from build123d import *

# Parameters (mm, degrees)
BOSS_EXTRU_1_START = -10
BOSS_EXTRU_1_DEPTH = 19
CHANFREIN1_SIZE    = 1.5


with BuildPart() as part:
    # Esquisse1 → Révolution1 (revolve)
    with BuildSketch(Plane.XY, mode=Mode.PRIVATE) as r_volution1_sk:
        Polygon((33, 0), (33, 35), (36, 41), (38.5, 41), (38.5, 42.25), (35.227457514, 42.25), (31.75, 35.295084972), (31.75, 0), align=None)
    revolve(r_volution1_sk.sketch.rotate(Axis((0, 0, 0), (0, 1, 0)), 90), axis=Axis((0, 0, 0), (0, 1, 0)))

    # Esquisse2 → Boss.-Extru.1 (add)
    with BuildSketch(Plane.XZ.offset(BOSS_EXTRU_1_START)):
        Polygon((-32.995416348, 0.55), (-36.495416348, 0.55), (-36.495416348, -0.55), (-32.995416348, -0.55), (-32.495416348, 0), align=None)
        Polygon((32.995416348, -0.55), (36.495416348, -0.55), (36.495416348, 0.55), (32.995416348, 0.55), (32.495416348, 0), align=None)
    extrude(amount=-BOSS_EXTRU_1_DEPTH)

    # Chanfrein1
    chanfrein1_edges = [part.edges().sort_by_distance(p)[0] for p in [
        (-36.495416348, 10, 0),
        (36.495416348, 10, 0),
    ]]
    chamfer(chanfrein1_edges, length=CHANFREIN1_SIZE)


solid = part.part
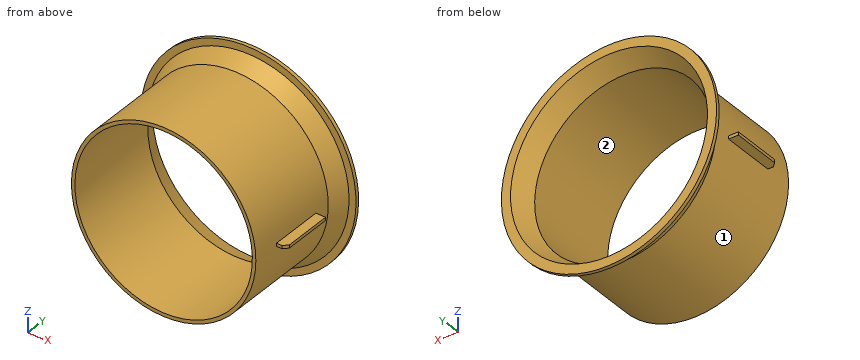
Design review of the part built by this model. Coordinates are the model's own, in mm. Face numbers are marked on the shaded views. Round coordinates to 2 decimals unless told otherwise and drop trailing zeros. Write each loop counter-clockwise with the first axis right and the second up, starting at its lowest first coordinate (ties: lowest second). Pieces come first, ordered by that corner, then holes. Notation, with made-up numbers: M -29.75,-5 L -20.75,-5 A23 ccw -20.75,25 Z; hole C -12.5,27.5 d5. An arc over 180 degrees is marked long. One line per item, written item: value. Start each with the question number.
1. Take a section at A-A on x = 0. State the section outline as (y, z) points, then the cut area to 3 significant figures.
2. Take a section at C-C on y = 9. State the section outline as (x, z) points.
3. Draft analysis for pull direction X (two halves, no side actions). For the marked faces 1 and 2, state which applies: pulls with the +X half, pulls with the -X half, needs draft (parallel to the pull), parting line crosses it, or undercut.
4. Clearance check with flat-ended pins moving along their axes: P1, Ø1.8, axis at x = -35.5, y = 19.5, coming from the +Z side; P2, Ø1, axis at x = 34.5, y = 16, coming from the -Z side; P3, Ø4, axis at y = 18.5, z = 21, coming from the +X side; P4, Ø2, axis at x = 23.5, z = -21, coming from the -Y side. State where each tip first meets the part, or that it passes through.
5. To check wall thickness, follow probe 1 along X at (y, z) = (19, 0); probe 2 along Z at (x, y) = (-11.5, 25); probe 3 along X at (y, z) = (22.5, -1). State the ranges of each line that lie inside material, in increasing order. Write a range as from..to.
Computed:
1. outline: M 0,-33 L 35,-33 L 41,-36 L 41,-38.5 L 42.25,-38.5 L 42.25,-35.23 L 35.3,-31.75 L 0,-31.75 Z; M 0,31.75 L 35.3,31.75 L 42.25,35.23 L 42.25,38.5 L 41,38.5 L 41,36 L 35,33 L 0,33 Z
1. area: 113 mm²
2. outline: C 0,0 d66; hole C 0,0 d63.5
3. face 1: parting line crosses it
3. face 2: undercut
4. P1: stops at z = 0.55
4. P2: stops at z = -0.55
4. P3: stops at x = 26.98
4. P4: stops at y = 0
5. probe 1: x = -36.5..-31.75, 31.75..36.5
5. probe 2: z = -30.93..-29.59, 29.59..30.93
5. probe 3: x = -32.98..-31.73, 31.73..32.98
